Source: CAD feature listing. Evaluate the final solid. Frame: model axes, mm. A direction names the side the tool comes from. Give positions to 0.01 mm unless a question says otherwise; leave off trailing zeros. Write each loop counter-clockwise with the first axis right and the second up, starting at its lowest first coordinate (ties: lowest second). Pieces come first, ordered by that corner, then holes. Notation, with made-up numbers: (-21.75, 9.25) -> (-4.75, 9.25) arc R24 cw to (-4.75, 44.25) -> close; hole circle Ø3 at (-38.5, -38.75). An arc over 180 degrees is marked (long way). Use one line per item in the form item = value. Start each with the question number.
(1) Set-up query: faces 1 (the face through (29.095, 19.161, -2.465)), 2 (the face through (-88.1, 148, -2.5)), 3 (the face through (100.3, -140.4, -2.5)), 4 (the face through (-95.46, 73.86, -2.46)). Return all of +Z, -Z, +X, -X, +Y, -Y with unobstructed straight access to the full face (end or side cutting, diameter ignored); none if empty.
(2) Cut plane B-B, the plane y = 139.5. Output: boundary loops of the cut face in (x, z).
(3) Draft query along X for faces 5 (the face through (2, 2, -5)), 6 (the face through (28.57, -18.79, -2.46)), 7 (the face through (-95.32, -74, -2.46)), 8 (the face through (95.46, -73.86, -2.46)). Return one class per face: pulls with the +X half, pulls with the -X half, needs draft (parallel to the pull), parting line crosses it, or undercut.
(4) Cut plane C-C, the plane y = -119.5. Output: boundary loops of the cut face in (x, z).
(5) Cut plane A-A, the plane y = -13. Output: boundary loops of the cut face in (x, z).
(6) First-contact query: P1, Ø1, axis at y = -44.5, z = -0.5, coming from the +X side; P2, Ø1.5, axis at y = 80.5, z = -1.5, coming from the -X side; P3, Ø2.5, axis at x = -19.5, z = -2.5, coming from the +Y side. Flat tips, straight axial feed; report the tip coordinate or a pass-through.
(7) Cut plane D-D, the plane z = -0.75. Count the separate pieces of the cut face and the enclosed holes in it, and give its area (3 significant figures).
(8) Material intervals for line 1 along Y through (x, z) = (75, -3.55); line 2 along Y through (x, z) = (0, -1.15); line 3 along Y through (x, z) = (-94.5, -0.8), sorted ascending. Write a range as from..to.
from build123d import *

# Parameters (mm, degrees)
SCHIZZO1_R                   = 1.25
ESTRUSIONE_ESTRUSIONE1_DEPTH = 5


with BuildPart() as part:
    # Schizzo1 → Estrusione-Estrusione1 (new body)
    with BuildSketch(Plane.XY):
        Polygon((-111.130864092, 156.55753287), (-106.55753287, 161.130864092), (-100.431262317, 160.330757253), (-75.393295673, 135.29279061), (75.393295673, 135.29279061), (100.431262317, 160.330757253), (106.55753287, 161.130864092), (111.130864092, 156.55753287), (110.330757253, 150.431262317), (90.448609444, 130.549114507), (90.448609444, 78.874114811), (100.330757253, 68.991967001), (100.330757253, 35.563826068), (90.448609444, 25.681678258), (90.448609444, -25.681678258), (100.330757253, -35.563826068), (100.330757253, -68.991967001), (90.448609444, -78.874114811), (90.448609444, -130.549114507), (110.330757253, -150.431262317), (111.130864092, -156.55753287), (106.55753287, -161.130864092), (100.431262317, -160.330757253), (75.393295673, -135.29279061), (-75.393295673, -135.29279061), (-100.431262317, -160.330757253), (-106.55753287, -161.130864092), (-111.130864092, -156.55753287), (-110.330757253, -150.431262317), (-90.448609444, -130.549114507), (-90.448609444, -78.874114811), (-100.330757253, -68.991967001), (-100.330757253, -35.563826068), (-90.448609444, -25.681678258), (-90.448609444, 21.125885189), (-100.330757253, 31.008032999), (-100.330757253, 68.991967001), (-90.448609444, 78.874114811), (-90.448609444, 130.549114507), (-110.330757253, 150.431262317), align=None)
        with Locations((-95, 50)):
            Circle(SCHIZZO1_R, mode=Mode.SUBTRACT)
        with Locations((-75, 50)):
            Circle(SCHIZZO1_R, mode=Mode.SUBTRACT)
        with Locations((-104.5, 154.5)):
            Circle(SCHIZZO1_R, mode=Mode.SUBTRACT)
        with Locations((104.5, 154.5)):
            Circle(SCHIZZO1_R, mode=Mode.SUBTRACT)
        with Locations((75, 50)):
            Circle(SCHIZZO1_R, mode=Mode.SUBTRACT)
        with Locations((95, 50)):
            Circle(SCHIZZO1_R, mode=Mode.SUBTRACT)
        with Locations((0, 20.131279802)):
            Circle(SCHIZZO1_R, mode=Mode.SUBTRACT)
        with Locations((0, -20.131279802)):
            Circle(SCHIZZO1_R, mode=Mode.SUBTRACT)
        with Locations((95, -50)):
            Circle(SCHIZZO1_R, mode=Mode.SUBTRACT)
        with Locations((75, -50)):
            Circle(SCHIZZO1_R, mode=Mode.SUBTRACT)
        with Locations((104.5, -154.5)):
            Circle(SCHIZZO1_R, mode=Mode.SUBTRACT)
        with Locations((-104.5, -154.5)):
            Circle(SCHIZZO1_R, mode=Mode.SUBTRACT)
        with Locations((-75, -50)):
            Circle(SCHIZZO1_R, mode=Mode.SUBTRACT)
        with Locations((-95, -50)):
            Circle(SCHIZZO1_R, mode=Mode.SUBTRACT)
        with BuildLine():
            Line((-66.435665908, 19.62934529), (-66.435665908, -19.62934529))
            Line((-66.435665908, -19.62934529), (-54.243131725, -32.22180516))
            Line((-54.243131725, -32.22180516), (-47.563810674, -32.22180516))
            Line((-47.563810674, -32.22180516), (-10.101900389, -5.729003291))
            ThreePointArc((-10.101900389, -5.729003291), (-9.48052072, -5.015427148), (-9.256694819, -4.096076524))
            Line((-9.256694819, -4.096076524), (-9.256694819, 4.096076524))
            ThreePointArc((-9.256694819, 4.096076524), (-9.48052072, 5.015427148), (-10.101900389, 5.729003291))
            Line((-10.101900389, 5.729003291), (-47.563810674, 32.22180516))
            Line((-47.563810674, 32.22180516), (-54.243131725, 32.22180516))
            Line((-54.243131725, 32.22180516), (-66.435665908, 19.62934529))
        make_face(mode=Mode.SUBTRACT)
        Polygon((-58.942185062, 100.139969228), (-58.942185062, 68.700211283), (-12.181822312, 35.631608635), (12.181822312, 35.631608635), (58.942185062, 68.700211283), (58.942185062, 100.139969228), (48.942185062, 110.139969228), (-48.942185062, 110.139969228), align=None, mode=Mode.SUBTRACT)
        with BuildLine():
            Line((-86.448609444, 35.007036896), (-83.551390556, 35.007036896))
            ThreePointArc((-83.551390556, 35.007036896), (-80.722963432, 36.178609771), (-79.551390556, 39.007036896))
            Line((-79.551390556, 39.007036896), (-79.551390556, 62.007036896))
            ThreePointArc((-79.551390556, 62.007036896), (-80.722963432, 64.835464021), (-83.551390556, 66.007036896))
            Line((-83.551390556, 66.007036896), (-86.448609444, 66.007036896))
            ThreePointArc((-86.448609444, 66.007036896), (-89.277036568, 64.835464021), (-90.448609444, 62.007036896))
            Line((-90.448609444, 62.007036896), (-90.448609444, 39.007036896))
            ThreePointArc((-90.448609444, 39.007036896), (-89.277036568, 36.178609771), (-86.448609444, 35.007036896))
        make_face(mode=Mode.SUBTRACT)
        with BuildLine():
            Line((86.448609444, 66.007036896), (83.551390556, 66.007036896))
            ThreePointArc((83.551390556, 66.007036896), (80.722963432, 64.835464021), (79.551390556, 62.007036896))
            Line((79.551390556, 62.007036896), (79.551390556, 39.007036896))
            ThreePointArc((79.551390556, 39.007036896), (80.722963432, 36.178609771), (83.551390556, 35.007036896))
            Line((83.551390556, 35.007036896), (86.448609444, 35.007036896))
            ThreePointArc((86.448609444, 35.007036896), (89.277036568, 36.178609771), (90.448609444, 39.007036896))
            Line((90.448609444, 39.007036896), (90.448609444, 62.007036896))
            ThreePointArc((90.448609444, 62.007036896), (89.277036568, 64.835464021), (86.448609444, 66.007036896))
        make_face(mode=Mode.SUBTRACT)
        with BuildLine():
            Line((47.563810674, 32.22180516), (10.101900389, 5.729003291))
            ThreePointArc((10.101900389, 5.729003291), (9.48052072, 5.015427148), (9.256694819, 4.096076524))
            Line((9.256694819, 4.096076524), (9.256694819, -4.096076524))
            ThreePointArc((9.256694819, -4.096076524), (9.48052072, -5.015427148), (10.101900389, -5.729003291))
            Line((10.101900389, -5.729003291), (47.563810674, -32.22180516))
            Line((47.563810674, -32.22180516), (54.243131725, -32.22180516))
            Line((54.243131725, -32.22180516), (66.435665908, -19.62934529))
            Line((66.435665908, -19.62934529), (66.435665908, 19.62934529))
            Line((66.435665908, 19.62934529), (54.243131725, 32.22180516))
            Line((54.243131725, 32.22180516), (47.563810674, 32.22180516))
        make_face(mode=Mode.SUBTRACT)
        with BuildLine():
            Line((-86.448609444, -66.007036896), (-83.551390556, -66.007036896))
            ThreePointArc((-83.551390556, -66.007036896), (-80.722963432, -64.835464021), (-79.551390556, -62.007036896))
            Line((-79.551390556, -62.007036896), (-79.551390556, -39.007036896))
            ThreePointArc((-79.551390556, -39.007036896), (-80.722963432, -36.178609771), (-83.551390556, -35.007036896))
            Line((-83.551390556, -35.007036896), (-86.448609444, -35.007036896))
            ThreePointArc((-86.448609444, -35.007036896), (-89.277036568, -36.178609771), (-90.448609444, -39.007036896))
            Line((-90.448609444, -39.007036896), (-90.448609444, -62.007036896))
            ThreePointArc((-90.448609444, -62.007036896), (-89.277036568, -64.835464021), (-86.448609444, -66.007036896))
        make_face(mode=Mode.SUBTRACT)
        Polygon((-48.942185062, -110.139969228), (48.942185062, -110.139969228), (58.942185062, -100.139969228), (58.942185062, -68.700211283), (12.181822312, -35.631608635), (-12.181822312, -35.631608635), (-58.942185062, -68.700211283), (-58.942185062, -100.139969228), align=None, mode=Mode.SUBTRACT)
        with BuildLine():
            Line((86.448609444, -35.007036896), (83.551390556, -35.007036896))
            ThreePointArc((83.551390556, -35.007036896), (80.722963432, -36.178609771), (79.551390556, -39.007036896))
            Line((79.551390556, -39.007036896), (79.551390556, -62.007036896))
            ThreePointArc((79.551390556, -62.007036896), (80.722963432, -64.835464021), (83.551390556, -66.007036896))
            Line((83.551390556, -66.007036896), (86.448609444, -66.007036896))
            ThreePointArc((86.448609444, -66.007036896), (89.277036568, -64.835464021), (90.448609444, -62.007036896))
            Line((90.448609444, -62.007036896), (90.448609444, -39.007036896))
            ThreePointArc((90.448609444, -39.007036896), (89.277036568, -36.178609771), (86.448609444, -35.007036896))
        make_face(mode=Mode.SUBTRACT)
    extrude(amount=-ESTRUSIONE_ESTRUSIONE1_DEPTH)


solid = part.part
Geometry says:
q1.face_1 = +Z, -Z
q1.face_2 = +Z, -Z, +Y
q1.face_3 = +Z, -Z, +X
q1.face_4 = +Z, -Z, -X
q2.outline = (-99.4, -5) -> (-79.6, -5) -> (-79.6, 0) -> (-99.4, 0) -> close; (79.6, -5) -> (99.4, -5) -> (99.4, 0) -> (79.6, 0) -> close
q3.face_5 = needs draft
q3.face_6 = undercut
q3.face_7 = pulls with the -X half
q3.face_8 = pulls with the +X half
q4.outline = (-90.45, -5) -> (90.45, -5) -> (90.45, 0) -> (-90.45, 0) -> close
q5.outline = (-90.45, -5) -> (-66.44, -5) -> (-66.44, 0) -> (-90.45, 0) -> close; (-20.38, -5) -> (20.38, -5) -> (20.38, 0) -> (-20.38, 0) -> close; (66.44, -5) -> (90.45, -5) -> (90.45, 0) -> (66.44, 0) -> close
q6.P1 = 100.33
q6.P2 = -90.45
q6.P3 = 135.29
q7.separate_pieces = 1
q7.enclosed_holes = 22
q7.area = 31,900 mm^2
q8.line_1 = -135.29..-51.25, -48.75..48.75, 51.25..135.29
q8.line_2 = -135.29..-110.14, -35.63..-21.38, -18.88..18.88, 21.38..35.63, 110.14..135.29
q8.line_3 = -154.4..-134.6, -74.82..-51.15, -48.85..-29.73, 25.18..48.85, 51.15..74.82, 134.6..154.4
